Design review of the part built by this model. Coordinates are the model's own, in mm. A direction names the side the tool comes from. Coordinates: 2 decimals unless noted, no trailing zeros. Order: outer loops, then holes, each group sorted by start corner. A loop starts at its lowest first (then second) coordinate and runs counter-clockwise, first axis right, second up. Notation, with made-up numbers: M 4,26.25 L 55,26.25 A12 ccw 55,40.25 Z; hole C -40,-20.5 d5. An arc over 180 degrees is marked long. Answer in a Markdown table with one row per item.
from build123d import *

# Parameters (mm, degrees)
EXTRUDED_BOSS_FRONT_PLANE_WING_DEPTH      = 10.16
EXTRUDED_BOSS_FRONT_PLANE_WING_DEPTH_BACK = 10.16
EXTRUDED_CUT_RIGHT_PLANE_WING_DEPTH       = 32.315223135
EXTRUDED_CUT_RIGHT_PLANE_WING_DEPTH_BACK  = 32.315223135
SKETCH3_W                                 = 18.542
SKETCH3_H                                 = 14.351
F_2X_0_2D_HOLES_D                         = 5.08
F_0_35D_HOLE_D                            = 8.89
INNER_CONNECTING_FILLET_R                 = 0.254
OUTTER_CONNECTING_FILLET_R                = 1.016


with BuildPart() as part:
    # Sketch2 → Extruded Boss Front Plane Wing (new, two sides: drawn at the far end of the back side and taken through both)
    with BuildSketch(Plane.XY.offset(-EXTRUDED_BOSS_FRONT_PLANE_WING_DEPTH_BACK)):
        with BuildLine():
            Line((-19.05, 0), (19.05, 0))
            Line((19.05, 0), (19.05, 5.08))
            Line((19.05, 5.08), (-19.05, 15.24))
            ThreePointArc((-19.05, 15.24), (-25.4, 8.89), (-19.05, 2.54))
            Line((-19.05, 2.54), (-19.05, 0))
        make_face()
    extrude(amount=EXTRUDED_BOSS_FRONT_PLANE_WING_DEPTH + EXTRUDED_BOSS_FRONT_PLANE_WING_DEPTH_BACK)

    # Sketch3 → Extruded Cut Right Plane Wing (cut, two sides: drawn at the far end of the back side and taken through both)
    with BuildSketch(Plane(origin=(0, 0, 0), x_dir=(0, 0, -1), z_dir=(1, 0, 0)).offset(-EXTRUDED_CUT_RIGHT_PLANE_WING_DEPTH_BACK)):
        with Locations((0, 8.0645)):
            Rectangle(SKETCH3_W, SKETCH3_H)
    extrude(amount=EXTRUDED_CUT_RIGHT_PLANE_WING_DEPTH + EXTRUDED_CUT_RIGHT_PLANE_WING_DEPTH_BACK, mode=Mode.SUBTRACT)

    # 2X 0.2D Holes (through all)
    with Locations(Plane.XY.offset(10.16)):
        with Locations((-19.05, 8.89)):
            Hole(F_2X_0_2D_HOLES_D / 2)

    # 0.35D Hole (through all)
    with Locations(Plane(origin=(0, 0.889, 0), x_dir=(1, 0, 0), z_dir=(0, 1, 0))):
        with Locations((-19.05, 0)):
            Hole(F_0_35D_HOLE_D / 2)

    # Inner Connecting Fillet
    inner_connecting_fillet_edges = [part.edges().sort_by_distance(p)[0] for p in [
        (19.05, 5.08, 9.7155),
        (0, 0.889, -9.271),
        (0, 0.889, 9.271),
        (19.05, 5.08, -9.7155),
    ]]
    fillet(inner_connecting_fillet_edges, radius=INNER_CONNECTING_FILLET_R)

    # Outter Connecting Fillet
    outter_connecting_fillet_edges = [part.edges().sort_by_distance(p)[0] for p in [
        (0, 0, 10.16),
        (0, 0, -10.16),
    ]]
    fillet(outter_connecting_fillet_edges, radius=OUTTER_CONNECTING_FILLET_R)


solid = part.part
(1) Add section A-A, the plane y = 3.25. Give the boundary of the cut face in (x, z).
Return value:
| item | result |
|---|---|
| outline | M -21.97,-10.16 L 19.05,-10.16 L 19.05,-9.27 L -21.97,-9.27 Z; M -21.97,9.27 L 19.05,9.27 L 19.05,10.16 L -21.97,10.16 Z |
(2) For faces 5 (the flat face through (-19.05, 0.7, 7.9)), 6 (the flat face through (-3, 7, 9.271)), 7 (the flat face through (19.05, 0.6, -2.3)), list the 3-axis set-ups (+Z, -Z, +X, -X, +Y, -Y) from which the entire face can be reached by the end or side of a thin tool; tool diameter is ignored.
Return value:
| item | result |
|---|---|
| face 5 | +Z, -Z, -X, -Y |
| face 6 | +X, -X, +Y |
| face 7 | +Z, -Z, +X, +Y, -Y |
(3) Draft analysis for pull direction Z (two halves, no side actions). For faces 1 (the flat face through (-8, 7, -10.16)), 2 (the flat face through (0.171, 10.114, -9.722)), 3 (the flat face through (-3, 7, -9.271)), 4 (the cylindrical face through (-14.606, 0.438, -0.098)), state which applies: pulls with the +Z half, pulls with the -Z half, needs draft (parallel to the pull), parting line crosses it, or undercut.
Return value:
| item | result |
|---|---|
| face 1 | pulls with the -Z half |
| face 2 | needs draft |
| face 3 | undercut |
| face 4 | undercut |
(4) Add section C-C, the plane z = 0. Give the boundary of the cut face in (x, y) (3 decimals), and give its area (3 significant figures).
Return value:
| item | result |
|---|---|
| outline | M -14.605,0 L 19.05,0 L 19.05,0.889 L -14.605,0.889 Z |
| area | 29.9 mm2 |
(5) Add section D-D, the plane y = 9.75. Give the boundary of the cut face in (x, z), and give its area (3 significant figures).
Return value:
| item | result |
|---|---|
| outline | M -25.34,-10.16 L -21.44,-10.16 L -21.44,-9.27 L -25.34,-9.27 Z; M -25.34,9.27 L -21.44,9.27 L -21.44,10.16 L -25.34,10.16 Z; M -16.66,-10.16 L 1.54,-10.16 L 1.54,-9.27 L -16.66,-9.27 Z; M -16.66,9.27 L 1.54,9.27 L 1.54,10.16 L -16.66,10.16 Z |
| area | 39.3 mm2 |
(6) For line 1 along Z through (x, y) = (-6.5, 9.75); line 2 along X through (y, z) = (0.5, -5); line 3 along Y through (x, z) = (-5.5, 4), list the stretches that pass through material, from the lowest coordinate up. Write a range as from..to.
Return value:
| item | result |
|---|---|
| line 1 | z = -10.16..-9.27, 9.27..10.16 |
| line 2 | x = -19.05..19.05 |
| line 3 | y = 0..0.89 |
(7) Insertion check: pin 1 Ø2 at (y, z) = (1.5, 6.5) entering from -X; pin 2 Ø2 at (y, z) = (13.5, -8) entering from +X; pin 3 Ø1.5 at (x, z) = (12.5, -3.5) entering from +Y. Each pin has a flat end and moves straight along its axis. Give the tip position at first contact, or say it passes through.
Return value:
| item | result |
|---|---|
| pin 1 | stops at x = -19.05 |
| pin 2 | passes through |
| pin 3 | stops at y = 0.89 |
(8) Add section B-B, the plane y = 7.75. Give the boundary of the cut face in (x, z).
Return value:
| item | result |
|---|---|
| outline | M -25.3,-10.16 L -21.32,-10.16 L -21.32,-9.27 L -25.3,-9.27 Z; M -25.3,9.27 L -21.32,9.27 L -21.32,10.16 L -25.3,10.16 Z; M -16.78,-10.16 L 9.04,-10.16 L 9.04,-9.27 L -16.78,-9.27 Z; M -16.78,9.27 L 9.04,9.27 L 9.04,10.16 L -16.78,10.16 Z |
